from build123d import *

# Parameters (mm, degrees)
F0_W     = 4.3434
F0_H     = 12.7
F0_W_2   = 12.7
F0_H_2   = 4.3434
F1_DEPTH = 4.3434
F2_W     = 12.7
F2_H     = 4.3434
F3_DEPTH = 4.3444


with BuildPart() as f1:
    # F0 (on Right) → F1 (new body)
    with BuildSketch(Plane.YZ):
        Polygon((111.924825, 79.89284), (-53.175175, 79.89284), (-53.175175, 39.269085), (-53.175175, 26.569085), (-53.175175, -47.10716), (23.024825, -47.10716), (23.024825, -42.76376), (35.724825, -42.76376), (35.724825, -47.10716), (111.924825, -47.10716), (111.924825, 26.569085), (111.924825, 39.269085), align=None)
        with Locations((-55.346875, 32.919085)):
            Rectangle(F0_W, F0_H)
        with Locations((114.096525, 32.919085)):
            Rectangle(F0_W, F0_H)
        with Locations((29.374825, -44.93546)):
            Rectangle(F0_W_2, F0_H_2)
    extrude(amount=-F1_DEPTH)

    # F2 (on Right) → F3 (cut, through all)
    with BuildSketch(Plane.YZ):
        with Locations((29.374825, -44.93546)):
            Rectangle(F2_W, F2_H)
    extrude(amount=-F3_DEPTH, mode=Mode.SUBTRACT)


solid = f1.part
Check sheet for the modelled part. Datum: model origin and axes. Units: mm. A direction names the side the tool comes from. Give positions to 0.01 mm unless a question says otherwise; leave off trailing zeros. Loops run counter-clockwise (first coordinate to the right, second up) from the corner with the lowest first, then second, coordinate; pieces in that order, holes last. Notation, with made-up numbers: M 71,70.5 L 90,70.5 A18 ccw 90,80.5 Z; hole C -13.75,42 d10. An arc over 180 degrees is marked long. Use a Markdown table: item, result. Add a question column.
Q1. Go/stop test with flat-tipped pins: pin 1 (2 mm diameter, centred on x = -1, z = 2.5, fed in from -Y); pin 2 (2 mm diameter, centred on x = -2.5, z = 52, fed in from +Y); pin 3 (1.3 mm diameter, centred on x = -1.5, y = 28, fed in from -Z). Record where each tip stops, or that it passes through.
Q2. Scan line: line 1 along Y through (x, z) = (-2.75, 40). Record every from-to range of solid material in increasing order. Write a range as [from, to].
Q3. Tool access check on faces 1 (the flat face through (-2, 111.925, 59)), 2 (the flat face through (-2, -55, 39.269)), 3 (the flat face through (-2, -55, 26.569)), 4 (the flat face through (-2, 114, 26.569)). Record the directions out of +Z, -Z, +X, -X, +Y, -Y that give a thin tool (end or side, any length) a straight path to the whole face; none if there is none.
Q4. Sectioned sample at B-B, the plane z = 52. Record the cut outline in (x, y), then the cut area to 3 significant figures.
Q5. Mould release check, pull along Y, two halves, no side actions. Record for faces 5 (the flat face through (-2, 35.725, -45)), 6 (the flat face through (0, 28, 17)), 7 (the flat face through (-2, 111.925, -11)), 8 (the flat face through (-2, -53.175, -10)): pulls with the +Y half, pulls with the -Y half, needs draft (parallel to the pull), parting line crosses it, or undercut.
Q6. Sectioned sample at A-A, the plane x = -2.45. Record the cut outline in (y, z).
Verdict:
| question | item | result |
|---|---|---|
| 1 | pin 1 | y = -53.18 |
| 1 | pin 2 | y = 111.92 |
| 1 | pin 3 | z = -42.76 |
| 2 | line 1 | [-53.18, 111.92] |
| 3 | face 1 | +Z, +X, -X, +Y |
| 3 | face 2 | +Z, +X, -X, -Y |
| 3 | face 3 | -Z, +X, -X, -Y |
| 3 | face 4 | -Z, +X, -X, +Y |
| 4 | outline | M -4.34,-53.18 L 0,-53.18 L 0,111.92 L -4.34,111.92 Z |
| 4 | area | 717 mm^2 |
| 5 | face 5 | undercut |
| 5 | face 6 | needs draft |
| 5 | face 7 | pulls with the +Y half |
| 5 | face 8 | pulls with the -Y half |
| 6 | outline | M -57.52,26.57 L -53.18,26.57 L -53.18,-47.11 L 23.02,-47.11 L 23.02,-42.76 L 35.72,-42.76 L 35.72,-47.11 L 111.92,-47.11 L 111.92,26.57 L 116.27,26.57 L 116.27,39.27 L 111.92,39.27 L 111.92,79.89 L -53.18,79.89 L -53.18,39.27 L -57.52,39.27 Z |
